Geometry check sheet. Reference: drawing and pictorial views, mm from the part's lowest x, y, z. Give positions to 0.01 mm unless a question says otherwise; leave off trailing zeros. Loops run counter-clockwise (first coordinate to the right, second up) from the corner with the lowest first, then second, coordinate; pieces in that order, holes last. Notation, with made-up numbers: (47.5, 74) - (53.5, 74) arc R18 cw to (53.5, 79) - close; hole circle Ø11 at (30.25, 33). An arc over 180 degrees is marked (long way). Answer in a Markdown table with one row per item. Add a question column.
(1) Go/stop test with a flat-tipped pin: P1, Ø1.9, axis at x = 27.25, z = 2.75, coming from the +Y side. Record where the tip stops, or that it passes through.
(2) Thickness scan on L1, parallel to X at y = 0.5, z = 2.75; L2, parallel to Z at x = 28, y = 0.5. Record the ranges inside material, lowest first.
(3) Sectioned sample at A-A on y = 0.4. Enter the section's corners in (x, z), then the cut area to 3 significant figures.
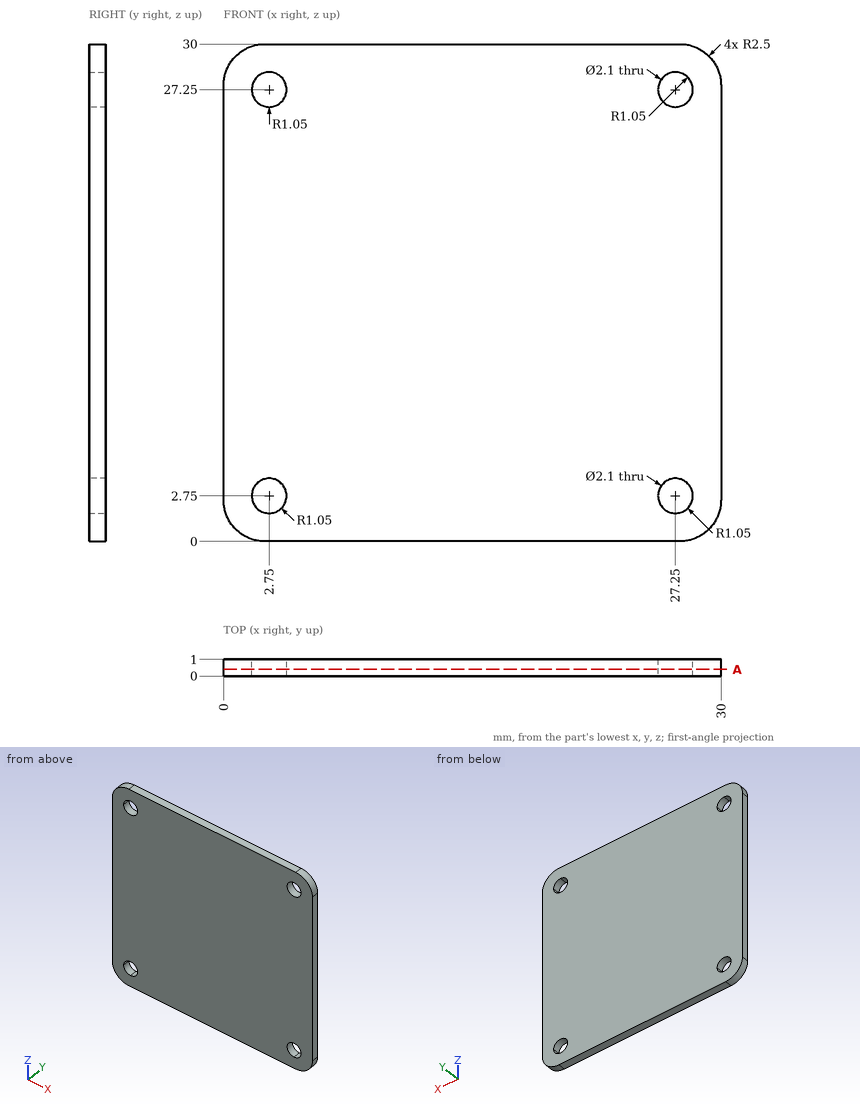
Reply:
| question | item | result |
|---|---|---|
| 1 | P1 | through |
| 2 | L1 | 0 to 1.7, 3.8 to 26.2, 28.3 to 30 |
| 2 | L2 | 0.05 to 2.02, 3.48 to 26.52, 27.98 to 29.95 |
| 3 | outline | (0, 2.5) arc R2.5 ccw to (2.5, 0) - (27.5, 0) arc R2.5 ccw to (30, 2.5) - (30, 27.5) arc R2.5 ccw to (27.5, 30) - (2.5, 30) arc R2.5 ccw to (0, 27.5) - close; hole circle Ø2.1 at (2.75, 2.75); hole circle Ø2.1 at (2.75, 27.25); hole circle Ø2.1 at (27.25, 2.75); hole circle Ø2.1 at (27.25, 27.25) |
| 3 | area | 881 mm^2 |
